Part print with two shaded views. Sizes in mm from the minimum x, y, z corner. A direction names the side the tool comes from. Round coordinates to 2 decimals unless told otherwise and drop trailing zeros. Write each loop counter-clockwise with the first axis right and the second up, starting at its lowest first coordinate (ties: lowest second). Pieces come first, ordered by that corner, then holes.
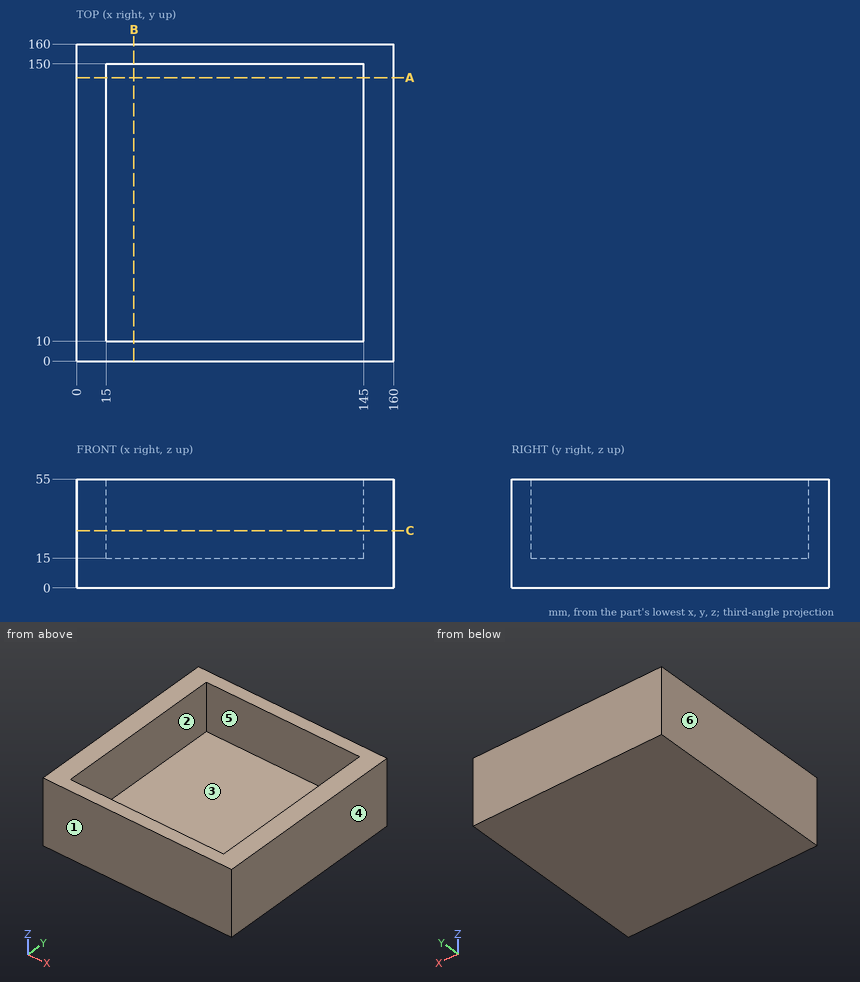
Q1. Wall check: L1, parallel to X at y = 42, z = 30; L2, parallel to Y at x = 27.5, z = 19.5; L3, parallel to Z at x = 101, y = 16.5. Give the ranges that are in metal, low to high.
Values follow:
L1: x = 0 to 15, 145 to 160
L2: y = 0 to 10, 150 to 160
L3: z = 0 to 15
Q2. Cut at B-B on x = 29. Write the cut outline in (y, z), plus the area to 3 significant figures.
Values follow:
outline: (0, 0) - (160, 0) - (160, 55) - (150, 55) - (150, 15) - (10, 15) - (10, 55) - (0, 55) - close
area: 3,200 mm2
Q3. Cut at C-C on z = 29. Write the cut outline in (x, y), plus the area to 3 significant figures.
Values follow:
outline: (0, 0) - (160, 0) - (160, 160) - (0, 160) - close; hole (15, 10) - (145, 10) - (145, 150) - (15, 150) - close
area: 7,400 mm2
Q4. Mould opens along X. For the marked faces 1, 2, 3 and 4 say: +X half, -X half, draft (parallel to the pull), parting line (faces both ways), or undercut.
Values follow:
face 1: draft
face 2: undercut
face 3: undercut
face 4: +X half
Q5. Which spindle directions (+Z, -Z, +X, -X, +Y, -Y) get a long thin tool onto all of the face, cutting with end or side? Do the marked faces 5 and 6. Say none if no direction does.
Values follow:
face 5: +Z
face 6: +Z, -Z, -X, +Y, -Y
Q6. Cut at A-A on y = 143. Write the cut outline in (x, z).
Values follow:
outline: (0, 0) - (160, 0) - (160, 55) - (145, 55) - (145, 15) - (15, 15) - (15, 55) - (0, 55) - close
